Here's the drawing with two shaded views (mm, measured from the low corner). I have some questions. A direction names the side the tool comes from. Give positions to 0.01 mm unless a question says otherwise; leave off trailing zeros. Order: outer loops, then holes, each group sorted by start corner. A loop starts at its lowest first (then second) coordinate and runs counter-clockwise, first axis right, second up. Notation, with made-up numbers: (62, 76.5) - (69, 76.5) arc R31 ccw to (69, 104.5) - close; hole circle Ø9 at (-16.5, -9). An arc over 180 degrees is marked (long way). Use one line per item in the form item = value. Start each with the question number.
1) Which directions (+Z, -Z, +X, -X, +Y, -Y) give clear straight access to the entire face, cutting with the end or side of a thin tool? Please do the marked faces 1 and 2.
2) For pin 1 (12 mm diameter, centred on y = 15, z = 35.5, fed in from -X); pin 2 (1.6 mm diameter, centred on y = 2, z = 61.5, fed in from +X) (1 decimal); pin 3 (20.5 mm diameter, centred on x = 16, y = 7.5, fed in from +Z) (1 decimal); pin 4 (3.5 mm diameter, centred on y = 2, z = 60, fed in from -X) (1 decimal), each with a flat end and sliding along its axis, tell me the tip position at first contact or that it passes through.
3) Please list where these lines run through material, in increasing order: probe 1 along Z at (x, y) = (8.5, 3.5) (1 decimal); probe 2 along Z at (x, y) = (79.5, 45.5) (1 decimal).
4) We'd pull the mould along X, two halves only. Please class the marked faces 3, 4 and 5: released by +X, released by -X, zero draft, split by the parting line, or undercut.
5) Suppose I cut it at A-A, the plane x = 47. Write out the boundary of the cut face in (y, z) (1 decimal).
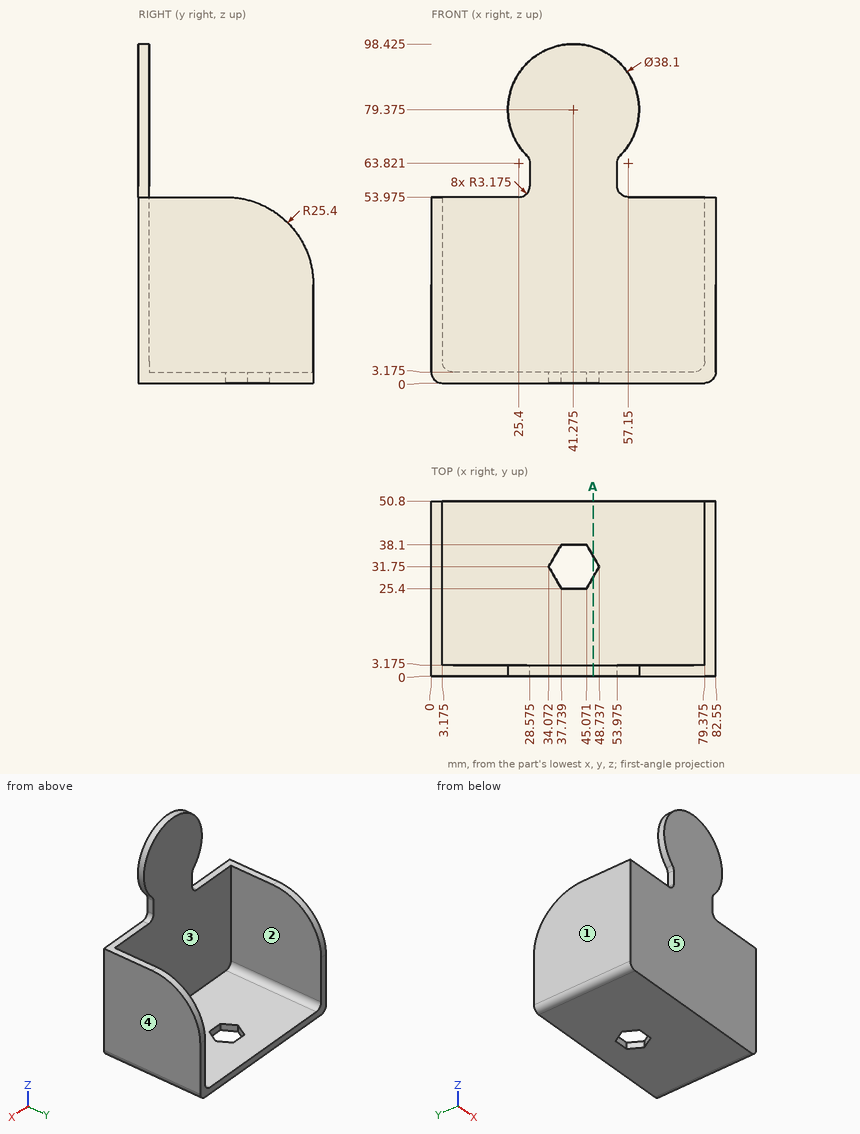
Result sheet:
q1.face_1 = +Z, -Z, -X, +Y, -Y
q1.face_2 = +Z, +Y
q2.pin_1 = 0
q2.pin_2 = 54
q2.pin_3 = 89.7
q2.pin_4 = 28.6
q3.probe_1 = 0 to 3.2
q3.probe_2 = 0 to 44.1
q4.face_3 = undercut
q4.face_4 = released by +X
q4.face_5 = zero draft
q5.outline = (0, 0) - (28.7, 0) - (28.7, 3.2) - (3.2, 3.2) - (3.2, 97.5) - (0, 97.5) - close; (34.8, 0) - (50.8, 0) - (50.8, 3.2) - (34.8, 3.2) - close
